```python
from build123d import *

# Parameters (mm, degrees)
SKETCH1_W           = 228.6
SKETCH1_H           = 228.6
SKETCH1_R           = 2.54
BOSS_EXTRUDE1_DEPTH = 2.54


with BuildPart() as part:
    # Sketch1 → Boss-Extrude1 (new body)
    with BuildSketch(Plane.XY):
        Rectangle(SKETCH1_W, SKETCH1_H)
        with Locations((-106.172, -106.172)):
            Circle(SKETCH1_R, mode=Mode.SUBTRACT)
        with BuildLine():
            Line((-3.81, -97.79), (-92.401846327, -97.79))
            Line((-92.401846327, -97.79), (-62.588329311, -67.976482983))
            ThreePointArc((-62.588329311, -67.976482983), (-35.360655709, -85.368174588), (-3.81, -92.323264158))
            Line((-3.81, -92.323264158), (-3.81, -97.79))
        make_face(mode=Mode.SUBTRACT)
        with BuildLine():
            ThreePointArc((-3.81, -84.696194523), (-32.444607955, -78.32821255), (-57.195176652, -62.583330324))
            Line((-57.195176652, -62.583330324), (-27.460573831, -32.848727503))
            ThreePointArc((-27.460573831, -32.848727503), (-16.384581274, -39.555878326), (-3.81, -42.645115942))
            Line((-3.81, -42.645115942), (-3.81, -84.696194523))
        make_face(mode=Mode.SUBTRACT)
        with BuildLine():
            Line((-67.976482983, -62.588329311), (-97.79, -92.401846327))
            Line((-97.79, -92.401846327), (-97.79, -3.81))
            Line((-97.79, -3.81), (-92.323264158, -3.81))
            ThreePointArc((-92.323264158, -3.81), (-85.368174588, -35.360655709), (-67.976482983, -62.588329311))
        make_face(mode=Mode.SUBTRACT)
        with BuildLine():
            ThreePointArc((-62.583330324, -57.195176652), (-78.32821255, -32.444607955), (-84.696194523, -3.81))
            Line((-84.696194523, -3.81), (-42.645115942, -3.81))
            ThreePointArc((-42.645115942, -3.81), (-39.555878326, -16.384581274), (-32.848727503, -27.460573831))
            Line((-32.848727503, -27.460573831), (-62.583330324, -57.195176652))
        make_face(mode=Mode.SUBTRACT)
        with BuildLine():
            Line((-3.81, -12.415847502), (-3.81, -34.988142381))
            ThreePointArc((-3.81, -34.988142381), (-13.46853352, -32.515916289), (-22.046275902, -27.434429575))
            Line((-22.046275902, -27.434429575), (-6.085253126, -11.473406799))
            ThreePointArc((-6.085253126, -11.473406799), (-4.970015818, -11.998679592), (-3.81, -12.415847502))
        make_face(mode=Mode.SUBTRACT)
        with BuildLine():
            ThreePointArc((-27.434429575, -22.046275902), (-32.515916289, -13.46853352), (-34.988142381, -3.81))
            Line((-34.988142381, -3.81), (-12.415847502, -3.81))
            ThreePointArc((-12.415847502, -3.81), (-11.998679592, -4.970015818), (-11.473406799, -6.085253126))
            Line((-11.473406799, -6.085253126), (-27.434429575, -22.046275902))
        make_face(mode=Mode.SUBTRACT)
        with BuildLine():
            ThreePointArc((3.81, -92.323264158), (35.360655709, -85.368174588), (62.588329311, -67.976482983))
            Line((62.588329311, -67.976482983), (92.401846327, -97.79))
            Line((92.401846327, -97.79), (3.81, -97.79))
            Line((3.81, -97.79), (3.81, -92.323264158))
        make_face(mode=Mode.SUBTRACT)
        with BuildLine():
            ThreePointArc((3.81, -42.645115942), (16.384581274, -39.555878326), (27.460573831, -32.848727503))
            Line((27.460573831, -32.848727503), (57.195176652, -62.583330324))
            ThreePointArc((57.195176652, -62.583330324), (32.444607955, -78.32821255), (3.81, -84.696194523))
            Line((3.81, -84.696194523), (3.81, -42.645115942))
        make_face(mode=Mode.SUBTRACT)
        with Locations((106.172, -106.172)):
            Circle(SKETCH1_R, mode=Mode.SUBTRACT)
        with BuildLine():
            ThreePointArc((3.81, -12.415847502), (4.970015818, -11.998679592), (6.085253126, -11.473406799))
            Line((6.085253126, -11.473406799), (22.046275902, -27.434429575))
            ThreePointArc((22.046275902, -27.434429575), (13.46853352, -32.515916289), (3.81, -34.988142381))
            Line((3.81, -34.988142381), (3.81, -12.415847502))
        make_face(mode=Mode.SUBTRACT)
        with BuildLine():
            Line((27.434429575, -22.046275902), (11.473406799, -6.085253126))
            ThreePointArc((11.473406799, -6.085253126), (11.998679592, -4.970015818), (12.415847502, -3.81))
            Line((12.415847502, -3.81), (34.988142381, -3.81))
            ThreePointArc((34.988142381, -3.81), (32.515916289, -13.46853352), (27.434429575, -22.046275902))
        make_face(mode=Mode.SUBTRACT)
        with BuildLine():
            Line((97.79, -92.401846327), (67.976482983, -62.588329311))
            ThreePointArc((67.976482983, -62.588329311), (85.368174588, -35.360655709), (92.323264158, -3.81))
            Line((92.323264158, -3.81), (97.79, -3.81))
            Line((97.79, -3.81), (97.79, -92.401846327))
        make_face(mode=Mode.SUBTRACT)
        with BuildLine():
            ThreePointArc((32.848727503, -27.460573831), (39.555878326, -16.384581274), (42.645115942, -3.81))
            Line((42.645115942, -3.81), (84.696194523, -3.81))
            ThreePointArc((84.696194523, -3.81), (78.32821255, -32.444607955), (62.583330324, -57.195176652))
            Line((62.583330324, -57.195176652), (32.848727503, -27.460573831))
        make_face(mode=Mode.SUBTRACT)
        with BuildLine():
            Line((-42.645115942, 3.81), (-84.696194523, 3.81))
            ThreePointArc((-84.696194523, 3.81), (-78.32821255, 32.444607955), (-62.583330324, 57.195176652))
            Line((-62.583330324, 57.195176652), (-32.848727503, 27.460573831))
            ThreePointArc((-32.848727503, 27.460573831), (-39.555878326, 16.384581274), (-42.645115942, 3.81))
        make_face(mode=Mode.SUBTRACT)
        with BuildLine():
            Line((-97.79, 3.81), (-97.79, 92.401846327))
            Line((-97.79, 92.401846327), (-67.976482983, 62.588329311))
            ThreePointArc((-67.976482983, 62.588329311), (-85.368174588, 35.360655709), (-92.323264158, 3.81))
            Line((-92.323264158, 3.81), (-97.79, 3.81))
        make_face(mode=Mode.SUBTRACT)
        with BuildLine():
            ThreePointArc((-34.988142381, 3.81), (-32.515916289, 13.46853352), (-27.434429575, 22.046275902))
            Line((-27.434429575, 22.046275902), (-11.473406799, 6.085253126))
            ThreePointArc((-11.473406799, 6.085253126), (-11.998679592, 4.970015818), (-12.415847502, 3.81))
            Line((-12.415847502, 3.81), (-34.988142381, 3.81))
        make_face(mode=Mode.SUBTRACT)
        with BuildLine():
            Line((-3.81, 34.988142381), (-3.81, 12.415847502))
            ThreePointArc((-3.81, 12.415847502), (-4.970015818, 11.998679592), (-6.085253126, 11.473406799))
            Line((-6.085253126, 11.473406799), (-22.046275902, 27.434429575))
            ThreePointArc((-22.046275902, 27.434429575), (-13.46853352, 32.515916289), (-3.81, 34.988142381))
        make_face(mode=Mode.SUBTRACT)
        with Locations((-106.172, 106.172)):
            Circle(SKETCH1_R, mode=Mode.SUBTRACT)
        with BuildLine():
            Line((-27.460573831, 32.848727503), (-57.195176652, 62.583330324))
            ThreePointArc((-57.195176652, 62.583330324), (-32.444607955, 78.32821255), (-3.81, 84.696194523))
            Line((-3.81, 84.696194523), (-3.81, 42.645115942))
            ThreePointArc((-3.81, 42.645115942), (-16.384581274, 39.555878326), (-27.460573831, 32.848727503))
        make_face(mode=Mode.SUBTRACT)
        with BuildLine():
            Line((-62.588329311, 67.976482983), (-92.401846327, 97.79))
            Line((-92.401846327, 97.79), (-3.81, 97.79))
            Line((-3.81, 97.79), (-3.81, 92.323264158))
            ThreePointArc((-3.81, 92.323264158), (-35.360655709, 85.368174588), (-62.588329311, 67.976482983))
        make_face(mode=Mode.SUBTRACT)
        with BuildLine():
            Line((0.020917227, -5.367236445), (0, -5.388153673))
            Line((0, -5.388153673), (-0.020917227, -5.367236445))
            ThreePointArc((-0.020917227, -5.367236445), (-2.053968063, -4.958717554), (-3.780418573, -3.81))
            Line((-3.780418573, -3.81), (-3.81, -3.81))
            Line((-3.81, -3.81), (-3.81, -3.780418573))
            ThreePointArc((-3.81, -3.780418573), (-4.958717554, -2.053968063), (-5.367236445, -0.020917227))
            Line((-5.367236445, -0.020917227), (-5.388153673, 0))
            Line((-5.388153673, 0), (-5.367236445, 0.020917227))
            ThreePointArc((-5.367236445, 0.020917227), (-4.958717554, 2.053968063), (-3.81, 3.780418573))
            Line((-3.81, 3.780418573), (-3.81, 3.81))
            Line((-3.81, 3.81), (-3.780418573, 3.81))
            ThreePointArc((-3.780418573, 3.81), (-2.053968063, 4.958717554), (-0.020917227, 5.367236445))
            Line((-0.020917227, 5.367236445), (0, 5.388153673))
            Line((0, 5.388153673), (0.020917227, 5.367236445))
            ThreePointArc((0.020917227, 5.367236445), (2.053968063, 4.958717554), (3.780418573, 3.81))
            Line((3.780418573, 3.81), (3.81, 3.81))
            Line((3.81, 3.81), (3.81, 3.780418573))
            ThreePointArc((3.81, 3.780418573), (4.958717554, 2.053968063), (5.367236445, 0.020917227))
            Line((5.367236445, 0.020917227), (5.388153673, 0))
            Line((5.388153673, 0), (5.367236445, -0.020917227))
            ThreePointArc((5.367236445, -0.020917227), (4.958717554, -2.053968063), (3.81, -3.780418573))
            Line((3.81, -3.780418573), (3.81, -3.81))
            Line((3.81, -3.81), (3.780418573, -3.81))
            ThreePointArc((3.780418573, -3.81), (2.053968063, -4.958717554), (0.020917227, -5.367236445))
        make_face(mode=Mode.SUBTRACT)
        with BuildLine():
            Line((34.988142381, 3.81), (12.415847502, 3.81))
            ThreePointArc((12.415847502, 3.81), (11.998679592, 4.970015818), (11.473406799, 6.085253126))
            Line((11.473406799, 6.085253126), (27.434429575, 22.046275902))
            ThreePointArc((27.434429575, 22.046275902), (32.515916289, 13.46853352), (34.988142381, 3.81))
        make_face(mode=Mode.SUBTRACT)
        with BuildLine():
            Line((22.046275902, 27.434429575), (6.085253126, 11.473406799))
            ThreePointArc((6.085253126, 11.473406799), (4.970015818, 11.998679592), (3.81, 12.415847502))
            Line((3.81, 12.415847502), (3.81, 34.988142381))
            ThreePointArc((3.81, 34.988142381), (13.46853352, 32.515916289), (22.046275902, 27.434429575))
        make_face(mode=Mode.SUBTRACT)
        with BuildLine():
            ThreePointArc((42.645115942, 3.81), (39.555878326, 16.384581274), (32.848727503, 27.460573831))
            Line((32.848727503, 27.460573831), (62.583330324, 57.195176652))
            ThreePointArc((62.583330324, 57.195176652), (78.32821255, 32.444607955), (84.696194523, 3.81))
            Line((84.696194523, 3.81), (42.645115942, 3.81))
        make_face(mode=Mode.SUBTRACT)
        with BuildLine():
            Line((97.79, 92.401846327), (97.79, 3.81))
            Line((97.79, 3.81), (92.323264158, 3.81))
            ThreePointArc((92.323264158, 3.81), (85.368174588, 35.360655709), (67.976482983, 62.588329311))
            Line((67.976482983, 62.588329311), (97.79, 92.401846327))
        make_face(mode=Mode.SUBTRACT)
        with BuildLine():
            Line((57.195176652, 62.583330324), (27.460573831, 32.848727503))
            ThreePointArc((27.460573831, 32.848727503), (16.384581274, 39.555878326), (3.81, 42.645115942))
            Line((3.81, 42.645115942), (3.81, 84.696194523))
            ThreePointArc((3.81, 84.696194523), (32.444607955, 78.32821255), (57.195176652, 62.583330324))
        make_face(mode=Mode.SUBTRACT)
        with BuildLine():
            ThreePointArc((62.588329311, 67.976482983), (35.360655709, 85.368174588), (3.81, 92.323264158))
            Line((3.81, 92.323264158), (3.81, 97.79))
            Line((3.81, 97.79), (92.401846327, 97.79))
            Line((92.401846327, 97.79), (62.588329311, 67.976482983))
        make_face(mode=Mode.SUBTRACT)
        with Locations((106.172, 106.172)):
            Circle(SKETCH1_R, mode=Mode.SUBTRACT)
    extrude(amount=BOSS_EXTRUDE1_DEPTH)


solid = part.part
```
The listing builds one solid part. Answer for the finished solid, in the listing's coordinates (mm). Coordinates: 2 decimals unless noted, no trailing zeros. Write each loop counter-clockwise with the first axis right and the second up, starting at its lowest first coordinate (ties: lowest second). Pieces come first, ordered by that corner, then holes. Notation, with made-up numbers: M 54,7.5 L 72,7.5 A23 ccw 72,15.5 Z; hole C 5,27 d11. An arc over 180 degrees is marked long. Use a Markdown table: item, result. Add a question column.
1. Section C-C (z = 2) is taken. Count the separate pieces of the cut face and the enclosed holes in it, plus the area to 3 significant figures.
2. Section B-B (x = -71.5) is taken. Give the vertices of the cut face in (y, z).
3. Straight lines are drawn through the part: line 1 along Y through (x, z) = (-63, 0.6); line 2 along X through (y, z) = (-97, 1); line 3 along X through (y, z) = (-104, 2.3). For each, find the intervals that lie inside material, in ascending order. Write a range as [from, to].
4. Section A-A (y = 48) is taken. Give the vertices of the cut face in (x, z).
Data:
| question | item | result |
|---|---|---|
| 1 | separate pieces | 1 |
| 1 | enclosed holes | 29 |
| 1 | area | 25,900 mm2 |
| 2 | outline | M -114.3,0 L -97.79,0 L -97.79,2.54 L -114.3,2.54 Z; M -76.89,0 L -66.11,0 L -66.11,2.54 L -76.89,2.54 Z; M -58.53,0 L -45.56,0 L -45.56,2.54 L -58.53,2.54 Z; M -3.81,0 L 3.81,0 L 3.81,2.54 L -3.81,2.54 Z; M 45.56,0 L 58.53,0 L 58.53,2.54 L 45.56,2.54 Z; M 66.11,0 L 76.89,0 L 76.89,2.54 L 66.11,2.54 Z; M 97.79,0 L 114.3,0 L 114.3,2.54 L 97.79,2.54 Z |
| 3 | line 1 | y = [-114.3, -97.79], [-68.39, -56.74], [-3.81, 3.81], [56.74, 68.39], [97.79, 114.3] |
| 3 | line 2 | x = [-114.3, -91.61], [-3.81, 3.81], [91.61, 114.3] |
| 3 | line 3 | x = [-114.3, -107.49], [-104.86, 104.86], [107.49, 114.3] |
| 4 | outline | M -114.3,0 L -97.79,0 L -97.79,2.54 L -114.3,2.54 Z; M -78.96,0 L -69.89,0 L -69.89,2.54 L -78.96,2.54 Z; M -53.39,0 L -42.61,0 L -42.61,2.54 L -53.39,2.54 Z; M -3.81,0 L 3.81,0 L 3.81,2.54 L -3.81,2.54 Z; M 42.61,0 L 53.39,0 L 53.39,2.54 L 42.61,2.54 Z; M 69.89,0 L 78.96,0 L 78.96,2.54 L 69.89,2.54 Z; M 97.79,0 L 114.3,0 L 114.3,2.54 L 97.79,2.54 Z |
